Source: CAD feature listing. Evaluate the final solid. Frame: model axes, mm. Give positions to 0.01 mm unless a question says otherwise; leave off trailing zeros. Write each loop counter-clockwise with the first axis right and the second up, starting at its lowest first coordinate (ties: lowest second). Pieces come first, ordered by that corner, then holes. Notation, with made-up numbers: M -8.5,-20.75 L 36.5,-20.75 A18 cw 36.5,10.25 Z; hole C 81,-9.5 d10. An arc over 180 degrees is marked long. Answer as a JSON object with one key per item and string values. Group by question number.
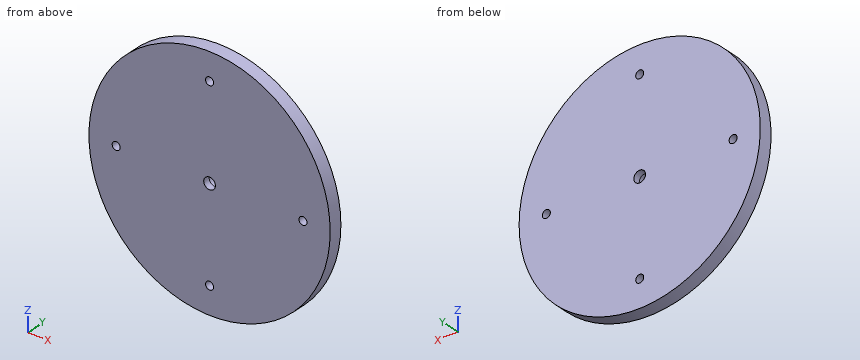
```python
from build123d import *

# Parameters (mm, degrees)
SKETCH1_R                = 98.425
SKETCH1_R_2              = 4.7625
BOSS_EXTRUDE1_DEPTH      = 5.55625
BOSS_EXTRUDE1_DEPTH_BACK = 5.55625
CIRPATTERN1_COUNT        = 4


with BuildPart() as part:
    # Sketch1 → Boss-Extrude1 (new body, two sides)
    with BuildSketch(Plane(origin=(0, 0, 0), x_dir=(1, 0, 0), z_dir=(0, 1, 0))) as boss_extrude1_sk:
        Circle(SKETCH1_R)
        Circle(SKETCH1_R_2, mode=Mode.SUBTRACT)
    extrude(amount=BOSS_EXTRUDE1_DEPTH)
    extrude(boss_extrude1_sk.sketch, amount=-BOSS_EXTRUDE1_DEPTH_BACK)

    # Sketch2 → 1/4 Clearance Hole1 (revolve, cut)
    with BuildSketch(Plane(origin=(0, 5.55625, 76.2), x_dir=(0, 0, 1), z_dir=(1, 0, 0))):
        Polygon((0, 0), (0, 14.661148974), (3.2639, 12.7), (3.2639, 0), align=None)
    f_1_4_clearance_hole1 = revolve(axis=Axis((0, 11.90625, 76.2), (0, -1, 0)), mode=Mode.SUBTRACT)

    # CirPattern1: 1/4 Clearance Hole1 ×4 about axis
    cirpattern1_axis = Axis((0, 0, 0), (0, 1, 0))
    for i in range(1, CIRPATTERN1_COUNT):
        add(f_1_4_clearance_hole1.rotate(cirpattern1_axis, i * 360 / CIRPATTERN1_COUNT), mode=Mode.SUBTRACT)


solid = part.part
```
(1) Section D-D, the plane z = -76.2. Return loops of the section in (x, y).
(2) Section C-C, the plane x = 76.2. Return loops of the section in (y, z).
(3) Contact query for flat-ended pins moving along their axis: pin 1 Ø6 at (x, z) = (0, -76.2) entering from +Y; pin 2 Ø3 at (x, y) = (-59.5, 3.5) entering from +Z; pin 3 Ø1 at (x, y) = (-16, 2) entering from -Z; pin 4 Ø3 at (x, y) = (-48.5, -0.5) entering from +Z. Output: stop coordinate, or through.
(4) Section A-A, the plane z = 0. Return loops of the section in (x, y) (1 decimal).
(5) Section B-B, the plane y = -3.75. State how many separate pieces and enclosed holes the cut face has, plus the area to 3 significant figures.
(6) Ray query, L1, parallel to X at y = -3, z = 3; L2, parallel to X at y = -1.5, z = -2; L3, parallel to Z at x = 76.2, y = -1. Return the intervals inside material, ascending. Write a range as [from, to].
Reported:
{
 "1": {"outline": "M -62.3,-5.56 L -3.26,-5.56 L -3.26,5.56 L -62.3,5.56 Z; M 3.26,-5.56 L 62.3,-5.56 L 62.3,5.56 L 3.26,5.56 Z"},
 "2": {"outline": "M -5.56,-62.3 L 5.56,-62.3 L 5.56,-3.26 L -5.56,-3.26 Z; M -5.56,3.26 L 5.56,3.26 L 5.56,62.3 L -5.56,62.3 Z"},
 "3": {"pin 1": "passes through", "pin 2": "stops at z = 79.52", "pin 3": "stops at z = -97.2", "pin 4": "stops at z = 86.48"},
 "4": {"outline": "M -98.4,-5.6 L -79.5,-5.6 L -79.5,5.6 L -98.4,5.6 Z; M -72.9,-5.6 L -4.8,-5.6 L -4.8,5.6 L -72.9,5.6 Z; M 4.8,-5.6 L 72.9,-5.6 L 72.9,5.6 L 4.8,5.6 Z; M 79.5,-5.6 L 98.4,-5.6 L 98.4,5.6 L 79.5,5.6 Z"},
 "5": {"separate pieces": "1", "enclosed holes": "5", "area": "30,200 mm2"},
 "6": {"L1": "x = [-98.38, -77.49], [-74.91, -3.7], [3.7, 74.91], [77.49, 98.38]", "L2": "x = [-98.4, -78.78], [-73.62, -4.32], [4.32, 73.62], [78.78, 98.4]", "L3": "z = [-62.3, -3.26], [3.26, 62.3]"}
}
